Autodesk Inventor part; units mm, degrees
ref_plane "YZ Plane" through (0, 0, 0) normal (1, 0, 0) x (0, 1, 0)
ref_plane "XZ Plane" through (0, 0, 0) normal (0, 1, 0) x (-1, 0, 0)
ref_plane "XY Plane" through (0, 0, 0) normal (0, 0, 1) x (1, 0, 0)
sketch "Эскиз3" plane through (0, 0, 0) normal (0, 1, 0) x (-1, 0, 0)
  arc A0 (1.791, 3.5766) -> (0.2774, -3.9904) centre (0, 0) ccw
  arc A1 (14, -18) -> (1.791, 3.5766) centre (-14.1884, -19.7077) ccw
  arc A2 (8, -18) -> (0.2774, -3.9904) centre (-13.2839, -20.5991) ccw
  line L0 (8, -18) -> (14, -18)
  line L1 (0, 0) -> (13.752, 0)
  dimension "d12" = 8
  dimension "d27" = 8
  dimension "d29" = 18
  dimension "d30" = 6
extrude "Выдавливание5" add sketch "Эскиз3" along normal blind 3
sketch "Эскиз5" plane through (0, 3, 0) normal (0, 1, 0) x (1, 0, 0)
  circle A0 centre (0, 0) radius 2
  dimension "d24" = 4
extrude "Выдавливание6" cut sketch "Эскиз5" against normal blind 10
mirror "Зеркальное отражение1" about plane through (-8, 0, -18) normal (0, 0, -1) of "Выдавливание5", "Выдавливание6"
properties part number "000.703 - Тяга" material "Пластик АБС"
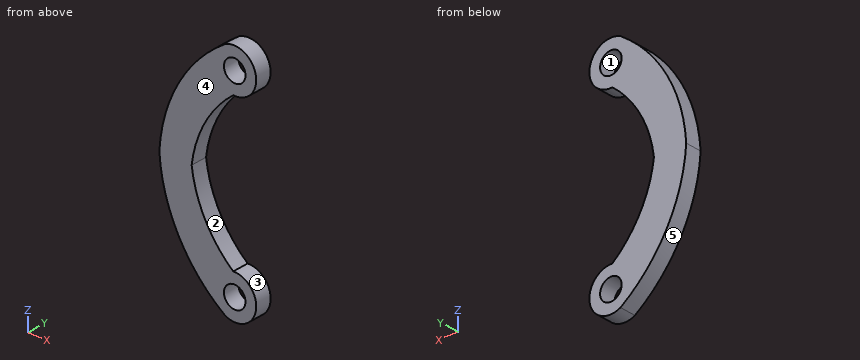
The listing builds one solid part. Answer for the finished solid, in the listing's coordinates (mm). Face numbers are marked on the shaded views. A direction names the side the tool comes from. Coordinates: 2 decimals unless noted, no trailing zeros. Loops run counter-clockwise (first coordinate to the right, second up) from the corner with the lowest first, then second, coordinate; pieces in that order, holes last. Notation, with made-up numbers: (-39.5, 81.5) -> (-24.5, 81.5) arc R17 cw to (-24.5, 88.5) -> close; hole circle Ø4 at (76, 65). An arc over 180 degrees is marked (long way). Return JSON: item names as keys, results as strings. Group by question number.
(1) A cutting plane is placed at D-D on x = -1. Write down the section's boundary in (y, z).
(2) A cutting plane is placed at A-A on x = -3. Write down the section's boundary in (y, z), and give its area (3 significant figures).
(3) Given pin 1 Ø3.5 at (x, z) = (0, -36) entering from -Y, flat-ended and moving along its own axis, determine where the tip first touches the part or whether it passes through.
(4) Find the intervals of material crossed by probe 1 along Z at (x, y) = (0, 1.5); probe 2 along Z at (x, y) = (1.75, 0.8); probe 3 along Z at (x, y) = (2.25, 1.1), in increasing order. Write a range as from..to.
(5) Determine the mould class of the marked faces 3, 4 and 5 for opening direction Z: released by +Z, released by -Z, zero draft, split by the parting line, or undercut.
(6) A cutting plane is placed at C-C on y = 1. Write down the section's boundary in (x, z), and give its area (3 significant figures).
(7) A cutting plane is placed at B-B on z = 0. Write down the section's boundary in (x, y), and give its area (3 significant figures).
(8) Which of the six approach directions +Z, -Z, +X, -X, +Y, -Y give full straight-line access (tool end or side, diameter ignored) to the marked faces 1 and 2?
The answers:
{
 "1": {"outline": "(0, -39.87) -> (3, -39.87) -> (3, -37.73) -> (0, -37.73) -> close; (0, -34.27) -> (3, -34.27) -> (3, -31.39) -> (0, -31.39) -> close; (0, -4.61) -> (3, -4.61) -> (3, -1.73) -> (0, -1.73) -> close; (0, 1.73) -> (3, 1.73) -> (3, 3.87) -> (0, 3.87) -> close"},
 "2": {"outline": "(0, -38.7) -> (3, -38.7) -> (3, -29.35) -> (0, -29.35) -> close; (0, -6.65) -> (3, -6.65) -> (3, 2.7) -> (0, 2.7) -> close", "area": "56.1 mm^2"},
 "3": {"pin 1": "passes through"},
 "4": {"probe 1": "z = -40..-38, -34..-32, -4..-2, 2..4", "probe 2": "z = -39.6..-36.97, -35.03..-32.4, -3.6..-0.97, 0.97..3.6", "probe 3": "z = -39.31..-32.69, -3.31..3.31"},
 "5": {"face 3": "undercut", "face 4": "zero draft", "face 5": "released by -Z"},
 "6": {"outline": "(-14, -18) arc R28.24 ccw to (-1.79, -39.58) arc R4 ccw (long way) to (-0.28, -32.01) arc R21.44 cw to (-8, -18) arc R21.44 cw to (-0.28, -3.99) arc R4 ccw (long way) to (-1.79, 3.58) arc R28.24 ccw to start; hole circle Ø4 at (0, -36); hole circle Ø4 at (0, 0)", "area": "313 mm^2"},
 "7": {"outline": "(-6.04, 0) -> (-2, 0) -> (-2, 3) -> (-6.04, 3) -> close; (2, 0) -> (4, 0) -> (4, 3) -> (2, 3) -> close", "area": "18.1 mm^2"},
 "8": {"face 1": "+Y, -Y", "face 2": "+X, +Y, -Y"}
}
